The drawing under review shows one solid part. Ordinate dimensions are in mm from its lowest x, y, z. Coordinates: 2 decimals unless noted, no trailing zeros. Write each loop counter-clockwise with the first axis right and the second up, starting at its lowest first coordinate (ties: lowest second). Pieces come first, ordered by that corner, then holes.
Q1. Insertion check: pin 1 (1 mm diameter, centred on x = 27, z = 3, fed in from -Y) (1 decimal); pin 2 (1 mm diameter, centred on x = 8, z = 2, fed in from -Y). Each pin has a flat end and moves straight along its axis. Give the tip position at first contact, or say it passes through.
Q2. Take a section at C-C (x = 32.5). Give the boundary of the cut face in (y, z).
Q3. Take a section at A-A (z = 2.05). Give the boundary of the cut face in (x, y), and give its area (3 significant figures).
Q4. For probe 1 along X at (y, z) = (17.75, 1) (1 decimal); probe 2 along X at (y, z) = (2.5, 2.65) (1 decimal); probe 3 along Y at (x, z) = (32, 0.45) (1 decimal), list the stretches that pass through material, from the lowest coordinate up.
Q5. Take a section at B-B (y = 11). Give the boundary of the cut face in (x, z), and give its area (3 significant figures).
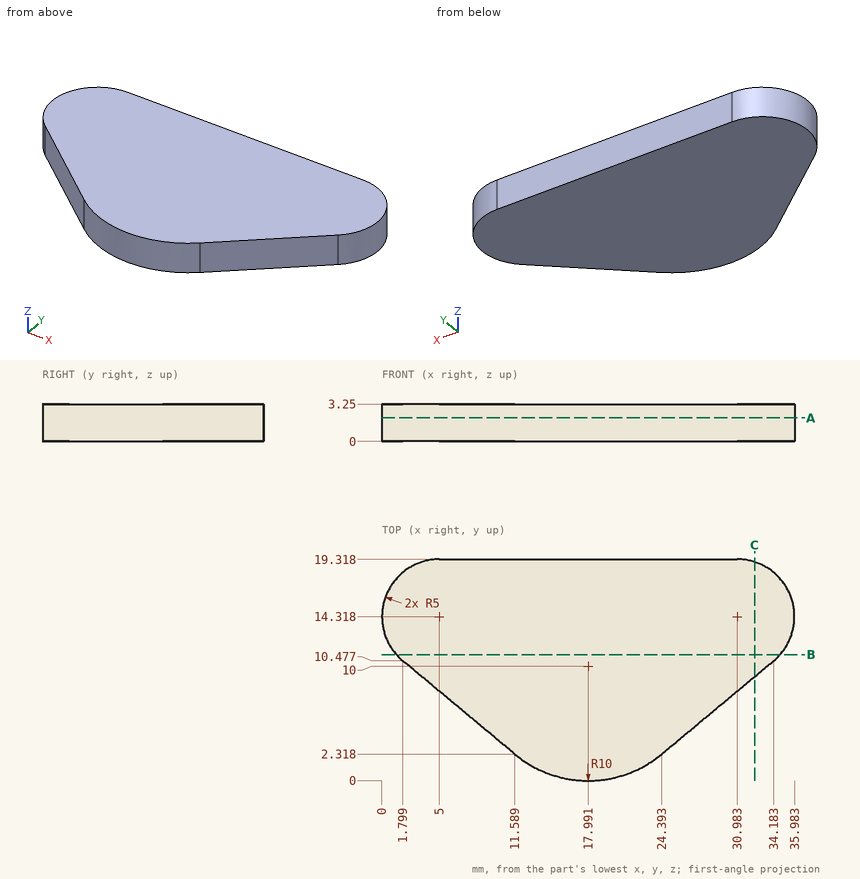
Response:
1. pin 1: stops at y = 4.1
1. pin 2: stops at y = 4.89
2. outline: (9.07, 0) - (19.08, 0) - (19.08, 3.25) - (9.07, 3.25) - close
3. outline: (1.8, 10.48) - (11.59, 2.32) arc R10 ccw to (24.39, 2.32) - (34.18, 10.48) arc R5 ccw to (30.98, 19.32) - (5, 19.32) arc R5 ccw to start
3. area: 508 mm2
4. probe 1: x = 1.4 to 34.6
4. probe 2: x = 11.4 to 24.6
4. probe 3: y = 8.7 to 19.2
5. outline: (1.26, 0) - (34.72, 0) - (34.72, 3.25) - (1.26, 3.25) - close
5. area: 109 mm2
